Input: part model. Units: mm. Frame: model coordinates. A direction names the side the tool comes from. Give positions to 0.01 mm unless a question says otherwise; leave off trailing zeros. Order: outer loops, then holes, each group sorted by start corner. A loop starts at its lowest first (then second) coordinate and runs counter-clockwise, first axis right, second up. Notation, with made-up numbers: (-32.5, 62.5) - (-20.5, 62.5) arc R17 cw to (-20.5, 89.5) - close; hole circle Ø7 at (89, 81). An arc over 180 degrees is marked (long way). Use a Markdown table: item, result.
Autodesk Inventor part; units mm, degrees
ref_plane "YZ Plane" through (0, 0, 0) normal (1, 0, 0) x (0, 1, 0)
ref_plane "XZ Plane" through (0, 0, 0) normal (0, 1, 0) x (-1, 0, 0)
ref_plane "XY Plane" through (0, 0, 0) normal (0, 0, 1) x (1, 0, 0)
sketch "Sketch1" plane through (0, 0, 0) normal (0, 1, 0) x (-1, 0, 0)
  line L0 (0, 0) -> (100.5, 0)
  line L1 (100.5, 0) -> (100.5, -165.5)
  line L2 (100.5, -165.5) -> (0, -165.5)
  line L3 (0, -165.5) -> (0, 0)
  line L4 (110.5, 2) -> (-13, 2)
  line L5 (-13, 2) -> (-13, -167.5)
  line L6 (-13, -167.5) -> (110.5, -167.5)
  line L7 (110.5, -167.5) -> (110.5, 2)
  line L8 (110.5, -157.5) -> (102.5, -157.5)
  line L9 (102.5, -157.5) -> (102.5, -8)
  line L10 (102.5, -8) -> (110.5, -8)
  line L11 (110.5, -8) -> (110.5, -157.5)
  line L12 (-13, -157.5) -> (-2, -157.5)
  line L13 (-2, -157.5) -> (-2, -8)
  line L14 (-2, -8) -> (-13, -8)
  line L15 (-13, -8) -> (-13, -157.5)
  point P0 (110.5, -8)
  point P1 (-13, -8)
  dimension "d0" = 100.5
  dimension "d1" = 165.5
  dimension "d2" = 2
  dimension "d3" = 13
  dimension "d4" = 10
  dimension "d5" = 2
  dimension "d33" = 8
  dimension "d34" = 8
  dimension "d35" = 8
  dimension "d36" = 8
  dimension "d37" = 2
  dimension "d38" = 2
extrude "Extrusion1" add sketch "Sketch1" against normal blind 8 contours L7 L10 L9 L8 L6 L5 L12 L13 L14 L4
sketch "Sketch2" plane through (0, 0, 0) normal (0, 1, 0) x (1, 0, 0)
  line L0 (-97, 3) -> (-8, 3)
  line L1 (-8, 3) -> (-8, 158.5)
  line L2 (-8, 158.5) -> (-97, 158.5)
  line L3 (-97, 158.5) -> (-97, 3)
  line L4 (-100.5, 0) -> (-100.5, 165.5)
  line L5 (-100.5, 165.5) -> (0, 165.5)
  line L6 (0, 165.5) -> (0, 0)
  line L7 (0, 0) -> (-100.5, 0)
  line L8 (13, -2) -> (-110.5, -2)
  line L9 (13, 167.5) -> (13, -2)
  line L10 (-110.5, -2) -> (13, -2)
  line L11 (13, -2) -> (13, 167.5)
  line L12 (13, 167.5) -> (-110.5, 167.5)
  line L13 (-110.5, 167.5) -> (-110.5, -2)
  dimension "d8" = 3.5
  dimension "d9" = 7
  dimension "d10" = 8
  dimension "d11" = 3
extrude "Extrusion2" add sketch "Sketch2" along normal blind 2 contours L4 L5 L6 L7 | L8 L13 L12 L9
sketch "Sketch3" plane through (0, -8, 0) normal (0, -1, 0) x (1, 0, 0)
  circle A0 centre (-106, -161.5) radius 1.75
  line L0 (-100.5, -165.5) -> (-100.5, 0)
  line L1 (0, -165.5) -> (-100.5, -165.5)
  circle A1 centre (-106, -4) radius 1.75
  line L2 (-100.5, 0) -> (0, 0)
  circle A2 centre (9.5, -4) radius 1.75
  line L3 (0, 0) -> (0, -165.5)
  circle A3 centre (9.5, -161.5) radius 1.75
  dimension "d14" = 3.5
  dimension "d15" = 5.5
  dimension "d16" = 4
  dimension "d17" = 3.5
  dimension "d18" = 4
  dimension "d19" = 5.5
  dimension "d20" = 3.5
  dimension "d21" = 4
  dimension "d22" = 9.5
  dimension "d23" = 3.5
  dimension "d24" = 9.5
  dimension "d25" = 4
extrude "Extrusion3" cut sketch "Sketch3" against normal blind 7 contours A0 | A1 | A2 | A3
chamfer "Chamfer1" distance 2 angle 45 4 edges at (-97, 2, -80.75) (-52.5, 2, -3) (-52.5, 2, -158.5) (-8, 2, -80.75)
equation "\"d14\" = hueco_diam"
equation "\"d17\" = hueco_diam"
equation "\"d20\" = hueco_diam"
equation "\"d21\" = hueco_sep_lat"
equation "\"d23\" = hueco_diam"
equation "\"d25\" = hueco_sep_lat"
equation "\"hueco_sep_inf\" = 4.5"
equation "\"hueco_sep_lat\" = 4"
equation "\"tol1\" = 0.5"
properties part number "PlantillaPantalla"
1. Section query D-D (x = -106). Return loops of the section in (y, z), then the cut area to 3 significant figures.
Response:
| item | result |
|---|---|
| outline | (-8, -167.5) - (2, -167.5) - (2, 2) - (-8, 2) - (-8, -2.25) - (-1, -2.25) - (-1, -5.75) - (-8, -5.75) - (-8, -8) - (0, -8) - (0, -157.5) - (-8, -157.5) - (-8, -159.75) - (-1, -159.75) - (-1, -163.25) - (-8, -163.25) - close |
| area | 450 mm^2 |
2. Mould query, pull axis X, two halves, no side actions, for faces 1 (the face through (-110.5, 0.4, -83.1)), 2 (the face through (-51, -4, -165.5)), 3 (the face through (-107, 0, -84)). Classes: pulls with the +X half, pulls with the -X half, needs draft (parallel to the pull), parting line crosses it, or undercut.
Response:
| item | result |
|---|---|
| face 1 | pulls with the -X half |
| face 2 | undercut |
| face 3 | needs draft |
3. Set-up query: faces 4 (the face through (-106, -4, -8)), 5 (the face through (8, -4, -157.5)), 6 (the face through (9, -1, -4)). Return all of +Z, -Z, +X, -X, +Y, -Y with unobstructed straight access to the full face (end or side cutting, diameter ignored); none if empty.
Response:
| item | result |
|---|---|
| face 4 | -X, -Y |
| face 5 | +X, -Y |
| face 6 | -Y |
4. Pin query (flat end, axial travel): pin 1 (5 mm diameter, centred on y = -5.5, z = -106, fed in from +X); pin 2 (3 mm diameter, centred on x = 9.5, z = -161.5, fed in from -Y); pin 3 (3.5 mm diameter, centred on x = 8.5, z = -105, fed in from -Y); pin 4 (4 mm diameter, centred on x = -106.5, z = -4.5, fed in from -Y). Return the tip coordinate at first contact, or that it passes through.
Response:
| item | result |
|---|---|
| pin 1 | stops at x = 2 |
| pin 2 | stops at y = -1 |
| pin 3 | stops at y = 0 |
| pin 4 | stops at y = -8 |
5. Material intervals for line 1 along X through (y, z) = (-4, -161.5); line 2 along Z through (x, y) = (9.5, -4.75); line 3 along X through (y, z) = (-5, -146.5), sorted ascending.
Response:
| item | result |
|---|---|
| line 1 | x = -110.5 to -107.75, -104.25 to -100.5, 0 to 7.75, 11.25 to 13 |
| line 2 | z = -167.5 to -163.25, -159.75 to -157.5, -8 to -5.75, -2.25 to 2 |
| line 3 | x = -102.5 to -100.5, 0 to 2 |
6. Section query C-C (y = -3). Return loops of the section in (x, z).
Response:
| item | result |
|---|---|
| outline | (-110.5, -167.5) - (13, -167.5) - (13, -157.5) - (2, -157.5) - (2, -8) - (13, -8) - (13, 2) - (-110.5, 2) - (-110.5, -8) - (-102.5, -8) - (-102.5, -157.5) - (-110.5, -157.5) - close; hole circle Ø3.5 at (-106, -161.5); hole circle Ø3.5 at (-106, -4); hole (-100.5, -165.5) - (0, -165.5) - (0, 0) - (-100.5, 0) - close; hole circle Ø3.5 at (9.5, -161.5); hole circle Ø3.5 at (9.5, -4) |
